Geometry check sheet. Reference: the model listing, model coordinates, mm. A direction names the side the tool comes from. Round coordinates to 2 decimals unless told otherwise and drop trailing zeros. Order: outer loops, then holes, each group sorted by start corner. A loop starts at its lowest first (then second) coordinate and runs counter-clockwise, first axis right, second up.
(1) Go/stop test with flat-tipped pins: pin 1 (4 mm diameter, centred on x = 298, z = 10, fed in from +Y); pin 2 (1.5 mm diameter, centred on x = 301, z = 12.5, fed in from +Y). Record where each tip stops, or that it passes through.
(2) Set-up check for faces 5 (the face through (296.5, 91, 10)), 6 (the face through (300, 91, 0)): record each of +Z, -Z, +X, -X, +Y, -Y from which the full face is reachable in a straight line by a thin tool's end or side.
(3) Sectioned sample at C-C (y = 90.85). Record the boundary of the cut face in (x, z).
(4) Material ranges on line 1 along X through (y, z) = (91, 8); line 2 along Z through (x, y) = (299.5, 90.35); line 3 along X through (y, z) = (90.1, 6.5), recorded low to high.
(5) Release check for a two-part mould opening along X. For faces 1 (the face through (296, 90, 10)), 2 (the face through (290.5, 91, 10)), 3 (the face through (299.9, 90.8, 5.7)), 4 (the face through (310.5, 91, 10)) record: +X half, -X half, draft (parallel to the pull), parting line (faces both ways), or undercut.
(6) Sectioned sample at A-A (z = 8.5). Record the boundary of the cut face in (x, y), plus the area to 3 significant figures.
(7) Sectioned sample at B-B (x = 303). Record the boundary of the cut face in (y, z), plus the area to 3 significant figures.
from build123d import *

# Parameters (mm, degrees)
BOX039_W          = 10
BOX039_H          = 10
BOX039_DEPTH      = 10
BOX040_W          = 10
BOX040_H          = 10
BOX040_DEPTH      = 10
CYLINDER030_R     = 4.3
CYLINDER030_DEPTH = 5
BOX041_W          = 20
BOX041_H          = 1.5
BOX041_DEPTH      = 20


with BuildPart() as cube039:
    # Box039 → Box039 (new body)
    with BuildSketch(Plane(origin=(53.5, -105, 4), x_dir=(1, 0, 0), z_dir=(0, 0, 1))):
        with Locations((5, 5)):
            Rectangle(BOX039_W, BOX039_H)
    extrude(amount=BOX039_DEPTH)


with BuildPart() as cube040:
    # Box040 → Box040 (new body)
    with BuildSketch(Plane(origin=(36.5, -105, 4), x_dir=(1, 0, 0), z_dir=(0, 0, 1))):
        with Locations((5, 5)):
            Rectangle(BOX040_W, BOX040_H)
    extrude(amount=BOX040_DEPTH)


with BuildPart() as cut047:
    # Cylinder030 → Cylinder030 (new body)
    with BuildSketch(Plane(origin=(50, -100, 9), x_dir=(1, 0, 0), z_dir=(0, -1, 0))):
        Circle(CYLINDER030_R)
    extrude(amount=CYLINDER030_DEPTH)

    # Cut046: cut Cube040
    add(cube040.part, mode=Mode.SUBTRACT)

    # Cut047: cut Cube039
    add(cube039.part, mode=Mode.SUBTRACT)


with BuildPart() as cut047_1:
    # Cut047 placement: moved
    add(cut047.part.moved(Location((250, 193, 1))))


with BuildPart() as obj1:
    # Box041 → Box041 (new body)
    with BuildSketch(Plane(origin=(290.5, 90, 0), x_dir=(1, 0, 0), z_dir=(0, 0, 1))):
        with Locations((10, 0.75)):
            Rectangle(BOX041_W, BOX041_H)
    extrude(amount=BOX041_DEPTH)

    # Cut048: cut Cut047
    add(cut047_1.part, mode=Mode.SUBTRACT)


solid = obj1.part
Answer below:
1. pin 1: stops at y = 91.5
1. pin 2: passes through
2. face 5: +Y, -Y
2. face 6: -Z, +X, -X, +Y, -Y
3. outline: (290.5, 0) - (310.5, 0) - (310.5, 20) - (290.5, 20) - close; hole (296.5, 7.5) arc R4.3 ccw to (303.5, 7.5) - (303.5, 12.5) arc R4.3 ccw to (296.5, 12.5) - close
4. line 1: x = 290.5 to 296.5, 303.5 to 310.5
4. line 2: z = 0 to 5.73, 14.27 to 20
4. line 3: x = 290.5 to 297.5, 302.5 to 310.5
5. face 1: draft
5. face 2: -X half
5. face 3: undercut
5. face 4: +X half
6. outline: (290.5, 90) - (296.5, 90) - (296.5, 91.5) - (290.5, 91.5) - close; (303.5, 90) - (310.5, 90) - (310.5, 91.5) - (303.5, 91.5) - close
6. area: 19.5 mm2
7. outline: (90, 0) - (91.5, 0) - (91.5, 6.92) - (90, 6.92) - close; (90, 13.08) - (91.5, 13.08) - (91.5, 20) - (90, 20) - close
7. area: 20.8 mm2
